from build123d import *

# Parameters (mm, degrees)
SKETCH1_W                        = 99.314
SKETCH1_H                        = 114.3
MAIN_DEPTH                       = 1.5875
SKETCH3_R                        = 46.0375
RAISED_DISK_EDGE_DEPTH           = 10.4775
SKETCH4_R                        = 44.45
DISK_HOLLOW_DEPTH                = 8.9375
SKETCH5_R                        = 1.905
SCREW_HOLES_ON_FRONT_PANEL_DEPTH = 2.54
SKETCH6_R                        = 3.81
SKETCH6_R_2                      = 1.2239625
MOUNTING_POSTS_DEPTH             = 17.4625
HOLLOW_REACH                     = 12.478
SKETCH8_R                        = 22.29794733


with BuildPart() as part:
    # Sketch1 → main (new body)
    with BuildSketch(Plane(origin=(0, 0, 0), x_dir=(1, 0, 0), z_dir=(0, 1, 0))):
        with Locations((-31.731304389, 36.593342839)):
            Rectangle(SKETCH1_W, SKETCH1_H)
    extrude(amount=MAIN_DEPTH)


with BuildPart() as body_2:
    # Sketch3 → raised disk edge (new body)
    with BuildSketch(Plane(origin=(0, 0, 0), x_dir=(1, 0, 0), z_dir=(0, 1, 0))):
        with Locations((-33.128304389, 27.068342839)):
            Circle(SKETCH3_R)
    extrude(amount=RAISED_DISK_EDGE_DEPTH)


with BuildPart() as disk_hollow_tool:
    # Sketch4 → disk hollow (new body, through all)
    with BuildSketch(Plane(origin=(0, 7.9375, 0), x_dir=(1, 0, 0), z_dir=(0, 1, 0))):
        with Locations((-33.128304389, 27.068342839)):
            Circle(SKETCH4_R)
    extrude(amount=-DISK_HOLLOW_DEPTH)


with BuildPart() as part_1:
    add(part.part)

    # disk hollow: cut by disk_hollow_tool
    add(disk_hollow_tool.part, mode=Mode.SUBTRACT)



with BuildPart() as body_2_1:
    add(body_2.part)

    # disk hollow: cut by disk_hollow_tool
    add(disk_hollow_tool.part, mode=Mode.SUBTRACT)

    # Sketch5 → screw holes on front panel (cut)
    with BuildSketch(Plane(origin=(0, 10.4775, 0), x_dir=(1, 0, 0), z_dir=(0, 1, 0))):
        with Locations((-33.128304389, 17.797342839)):
            Circle(SKETCH5_R)
        with Locations((-33.128304389, 5.478342839)):
            Circle(SKETCH5_R)
    extrude(amount=-SCREW_HOLES_ON_FRONT_PANEL_DEPTH, mode=Mode.SUBTRACT)


with BuildPart() as part_2:
    add(part_1.part)

    add(body_2_1.part)  # mounting posts merges body 2
    # Sketch6 → mounting posts (add)
    with BuildSketch(Plane(origin=(0, 1.5875, 0), x_dir=(1, 0, 0), z_dir=(0, 1, 0))):
        with Locations((-76.308304389, 2.303342839)):
            Circle(SKETCH6_R)
        with Locations((-76.308304389, 2.303342839)):
            Circle(SKETCH6_R_2, mode=Mode.SUBTRACT)
        with Locations((13.861695611, 22.623342839)):
            Circle(SKETCH6_R)
        with Locations((13.861695611, 22.623342839)):
            Circle(SKETCH6_R_2, mode=Mode.SUBTRACT)
        with Locations((-76.308304389, 88.663342839)):
            Circle(SKETCH6_R)
        with Locations((-76.308304389, 88.663342839)):
            Circle(SKETCH6_R_2, mode=Mode.SUBTRACT)
        with Locations((13.861695611, 88.663342839)):
            Circle(SKETCH6_R)
        with Locations((13.861695611, 88.663342839)):
            Circle(SKETCH6_R_2, mode=Mode.SUBTRACT)
    extrude(amount=MOUNTING_POSTS_DEPTH)

    # Sketch8 → hollow (cut, up to next)
    with BuildSketch(Plane(origin=(0, 10.4775, 0), x_dir=(1, 0, 0), z_dir=(0, 1, 0)), mode=Mode.PRIVATE) as hollow_sk1:
        with Locations((-33.128304389, 45.737342839)):
            Circle(SKETCH8_R)
    hollow_tool1 = extrude(hollow_sk1.sketch, amount=-HOLLOW_REACH, mode=Mode.PRIVATE) & part_2.part
    add(hollow_tool1.solids().sort_by_distance((-33.128304, 10.4775, -45.737343))[0], mode=Mode.SUBTRACT)


solid = part_2.part
Could you check a few things on this model? Use its own coordinates, in mm. A direction names the side the tool comes from. Give positions to 0.01 mm unless a question says otherwise; leave off trailing zeros. Order: outer loops, then holes, each group sorted by start corner. A loop starts at its lowest first (then second) coordinate and runs counter-clockwise, first axis right, second up. Notation, with made-up numbers: (71.5, 30) - (81.5, 30) arc R21 cw to (81.5, 56) - close; hole circle Ø5 at (59, -29.5). An arc over 180 degrees is marked (long way). One line per question, with ' | ' between items. Start each with the question number.
Item 1: I'm going to push flat-ended pins straight in: pin 1 Ø0.7 at (x, z) = (-76.5, -3) entering from +Y; pin 2 Ø1.5 at (y, z) = (3.5, -5) entering from +X; pin 3 Ø8 at (x, y) = (-2.5, 10.5) entering from -Z; pin 4 Ø3.5 at (x, z) = (-33.13, -5.48) entering from -Y. Where does each tip first touch, or does it pass through?
Item 2: Thinking about a two-plate mould opening in X: for faces 4 (the cylindrical face through (14.99, 10.2, -22.15)), 5 (the flat face through (-76.4, 19.05, -0.7)), which applies, pulls with the +X half, pulls with the -X half, needs draft (parallel to the pull), parting line crosses it, or undercut?
Item 3: I need wall thicknesses on probe 1 along X at (y, z) = (3.5, -1); probe 2 along Y at (x, z) = (-29.5, 9); probe 3 along X at (y, z) = (3, -50). Which ranges of each line are inside material? Lowest first, please. Write a range as [from, to].
Item 4: I want a section at A-A on y = 4.25. Give the number of separate pieces and of enclosed holes in the cut face, then the cut area to 3 significant figures.
Item 5: I want a section at D-D on y = 14.25. Write out the boundary of the cut face in (x, z).
Item 6: For faces 1 (the flat face through (-24, 7.938, -18)), 2 (the flat face through (-32, 1.588, -75)), 3 (the cylindrical face through (-31.31, 9.23, -6.05)), which set-ups out of +Z, -Z, +X, -X, +Y, -Y let a thin tool reach every point of the face, with its end or its side?
Item 7: I want a section at C-C on z = -52.5. Write out the boundary of the cut face in (x, y).
Item 8: I want a section at B-B on x = -20.5. Write out the boundary of the cut face in (y, z), then the cut area to 3 significant figures.
Verdict:
1) pin 1: y = 1.59 | pin 2: x = 7.68 | pin 3: z = -64.62 | pin 4: through
2) face 4: undercut | face 5: needs draft
3) probe 1: [-79.89, -72.73], [-71.07, -69.13], [2.88, 4.82] | probe 2: [7.94, 10.48] | probe 3: [-73.05, -71.21], [4.95, 6.79]
4) separate pieces: 3 | enclosed holes: 5 | area: 605 mm^2
5) outline: circle Ø7.62 at (-76.31, -88.66); circle Ø7.62 at (-76.31, -2.3); circle Ø7.62 at (13.86, -88.66); circle Ø7.62 at (13.86, -22.62); hole circle Ø2.45 at (-76.31, -88.66); hole circle Ø2.45 at (-76.31, -2.3); hole circle Ø2.45 at (13.86, -88.66); hole circle Ø2.45 at (13.86, -22.62)
6) face 1: -Y | face 2: +Y | face 3: +Y, -Y
7) outline: (-81.39, 0) - (-69.58, 0) - (-69.58, 7.94) - (-54.38, 7.94) - (-54.38, 10.48) - (-71.5, 10.48) - (-71.5, 1.59) - (-81.39, 1.59) - close; (-11.88, 7.94) - (3.33, 7.94) - (3.33, 0) - (17.93, 0) - (17.93, 1.59) - (5.25, 1.59) - (5.25, 10.48) - (-11.88, 10.48) - close
8) outline: (0, -93.74) - (1.59, -93.74) - (1.59, -71.34) - (10.48, -71.34) - (10.48, -64.11) - (7.94, -64.11) - (7.94, -69.69) - (0, -69.69) - close; (0, 15.55) - (7.94, 15.55) - (7.94, -27.36) - (10.48, -27.36) - (10.48, 17.2) - (1.59, 17.2) - (1.59, 20.56) - (0, 20.56) - close | area: 199 mm^2
